Design review of the part built by this model. Coordinates are the model's own, in mm. A direction names the side the tool comes from. Round coordinates to 2 decimals unless told otherwise and drop trailing zeros. Order: outer loops, then holes, each group sorted by start corner. A loop starts at its lowest first (then second) coordinate and runs counter-clockwise, first axis right, second up. Notation, with made-up numbers: (7, -37) - (62, -37) arc R18 cw to (62, -28) - close; hole circle Ø7 at (5.25, -37). An arc over 180 degrees is marked (long way). Write item = value, one per line.
from build123d import *

# Parameters (mm, degrees)
BOSS_EXTRUDE3_DEPTH = 2
BOSS_EXTRUDE4_DEPTH = 1
CUT_EXTRUDE4_DEPTH  = 1
CUT_EXTRUDE5_DEPTH  = 1
SKETCH7_W           = 100
SKETCH7_H           = 20.041590073
CUT_EXTRUDE6_DEPTH  = 166.541535573


with BuildPart() as part:
    # Sketch1 → Boss-Extrude3 (new body)
    with BuildSketch(Plane(origin=(0, 0, 0), x_dir=(1, 0, 0), z_dir=(0, 1, 0))):
        with BuildLine():
            Line((-50, 141.421356237), (-50, 50))
            Line((-50, 50), (0, 50))
            Line((0, 50), (43.299127574, 50))
            Line((43.299127574, 50), (50, 50))
            Line((50, 50), (50, 141.421356237))
            ThreePointArc((50, 141.421356237), (0, 150), (-50, 141.421356237))
        make_face()
        with BuildLine():
            Line((-70, 50), (-50, 50))
            Line((-50, 50), (-50, 141.421356237))
            ThreePointArc((-50, 141.421356237), (-60.159525267, 137.407538074), (-70, 132.664991614))
            Line((-70, 132.664991614), (-70, 50))
        make_face()
        Polygon((0, 50), (-50, 50), (-50, 29.958409927), (50, 29.958409927), (50, 50), (43.299127574, 50), align=None)
        with BuildLine():
            ThreePointArc((70, 132.664991614), (60.159525267, 137.407538074), (50, 141.421356237))
            Line((50, 141.421356237), (50, 50))
            Line((50, 50), (70, 50))
            Line((70, 50), (70, 132.664991614))
        make_face()
    extrude(amount=BOSS_EXTRUDE3_DEPTH)

    # Sketch2 → Boss-Extrude4 (add)
    with BuildSketch(Plane.XZ):
        with BuildLine():
            Line((50, -50), (-50, -50))
            Line((-50, -50), (-50, -141.421356237))
            ThreePointArc((-50, -141.421356237), (0, -150), (50, -141.421356237))
            Line((50, -141.421356237), (50, -50))
        make_face()
    extrude(amount=-BOSS_EXTRUDE4_DEPTH)

    # Sketch5 → Cut-Extrude4 (cut)
    with BuildSketch(Plane.XZ):
        with BuildLine():
            Line((-50, -141.421356237), (-50, -50))
            Line((-50, -50), (-70, -50))
            Line((-70, -50), (-70, -132.664991614))
            ThreePointArc((-70, -132.664991614), (-60.159525267, -137.407538074), (-50, -141.421356237))
        make_face()
    extrude(amount=-CUT_EXTRUDE4_DEPTH, mode=Mode.SUBTRACT)

    # Sketch6 → Cut-Extrude5 (cut)
    with BuildSketch(Plane.XZ):
        with BuildLine():
            ThreePointArc((50, -141.421356237), (60.159525267, -137.407538074), (70, -132.664991614))
            Line((70, -132.664991614), (70, -50))
            Line((70, -50), (50, -50))
            Line((50, -50), (50, -141.421356237))
        make_face()
    extrude(amount=-CUT_EXTRUDE5_DEPTH, mode=Mode.SUBTRACT)

    # Sketch7 → Cut-Extrude6 (cut, through all)
    with BuildSketch(Plane.XZ):
        with Locations((0, -39.979204964)):
            Rectangle(SKETCH7_W, SKETCH7_H)
    extrude(amount=-CUT_EXTRUDE6_DEPTH, mode=Mode.SUBTRACT)


solid = part.part
Item 1: Take a section at C-C, the plane x = -47.5. State the section outline as (y, z) points.
Data:
outline = (0, -142.28) - (2, -142.28) - (2, -50) - (0, -50) - close
Item 2: Take a section at B-B, the plane y = 1.3. State the section outline as (x, z) points (3 decimals).
Data:
outline = (-70, -132.665) arc R150 ccw to (70, -132.665) - (70, -50) - (-70, -50) - close
Item 3: For faces 1 (the face through (-60, 1, -95)), 2 (the face through (60, 1, -95)), 3 (the face through (-1, 0, -101)), list the 3-axis set-ups (+Z, -Z, +X, -X, +Y, -Y) from which the entire face can be reached by the end or side of a thin tool; tool diameter is ignored.
Data:
face_1 = +Z, -Z, -X, -Y
face_2 = +Z, -Z, +X, -Y
face_3 = +Z, -Z, +X, -X, -Y
Item 4: Insertion check: P1, Ø6, axis at x = 57, z = -104, coming from the -Y side; P2, Ø0.5, axis at y = 0.5, z = -92.5, coming from the -X side. Each pin has a flat end and moves straight along its axis. Give the tip position at first contact, or say it passes through.
Data:
P1 = 1
P2 = -50
Item 5: Take a section at D-D, the plane x = -23. State the section outline as (y, z) points.
Data:
outline = (0, -148.23) - (2, -148.23) - (2, -50) - (0, -50) - close
Item 6: Take a section at A-A, the plane z = -57. State the section outline as (x, y) points, and give its area (3 significant figures).
Data:
outline = (-70, 1) - (-50, 1) - (-50, 0) - (50, 0) - (50, 1) - (70, 1) - (70, 2) - (-70, 2) - close
area = 240 mm2
Item 7: For line 1 along X through (y, z) = (0.75, -77); line 2 along Y through (x, z) = (-61.5, -99.5); line 3 along Z through (x, y) = (-21.5, 1.55), list the stretches that pass through material, from the lowest coordinate up. Write a range as [from, to].
Data:
line_1 = [-50, 50]
line_2 = [1, 2]
line_3 = [-148.45, -50]
